Model file for the job. Use its own axes, mm. A direction names the side the tool comes from. Give positions to 0.01 mm unless a question says otherwise; leave off trailing zeros. Loops run counter-clockwise (first coordinate to the right, second up) from the corner with the lowest first, then second, coordinate; pieces in that order, holes last. Notation, with made-up numbers: M -2,23 L 38,23 A30 ccw 38,48 Z; hole C 50.25,-1.75 d8. An arc over 180 degrees is marked long. Use CSV: the item, a comma, the result in double quotes. Start each with the question number.
(1) Slice it at A-A on z = 20. State how many separate pieces and enclosed holes the cut face has, and give its area (3 significant figures).
(2) Wall check: line 1 along Y through (x, z) = (7, 2); line 2 along X through (y, z) = (11, 28); line 3 along Y through (x, z) = (0.7, 128.8). Give the ranges that are in metal, low to high. Write a range as from..to.
(3) Two-plate mould, pull along X, no slides. Class faces 1 (the face through (4, 7, 62)), 2 (the face through (37.14, 19.1, 1.52)), 3 (the face through (25.085, 15.049, 63.639)): pulls with the +X half, pulls with the -X half, needs draft (parallel to the pull), parting line crosses it, or undercut.
(4) Tool access for faces 4 (the face through (28.42, 6.35, 63.84)), 5 (the face through (6, 2, 3)), 6 (the face through (0.9, 19.14, 1.52)), 7 (the face through (12.724, 17.718, 62.16)): list every direction of +Z, -Z, +X, -X, +Y, -Y with a clear straight run to the whole face (end or side of a thin tool).
(5) Flat gauge pins, fed straight in: P1, Ø7.5, axis at x = 7, y = 4.5, coming from the +Z side; P2, Ø4, axis at x = 32, y = 29, coming from the -Z side; P3, Ø2.5, axis at y = -0.96, z = 128.8, coming from the +X side; P4, Ø1.5, axis at y = 3.5, z = 45.5, coming from the +X side. Where does each tip first touch, or does it go through?
(6) Slice it at B-B on y = 38.5. List the corners of the cut face in (x, z), and give its area (3 significant figures).
Autodesk Fusion 360 part; units mm, degrees
sketch "스케치1" plane through (0, 0, 0) normal (0, 0, 1) x (1, 0, 0)
  line L0 (0, 0) -> (38, 0)
  line L1 (38, 0) -> (38, 20)
  line L2 (38, 20) -> (0, 20)
  line L3 (0, 20) -> (0, 0)
  line L4 (0, 0) -> (0, 10)
  circle A0 centre (7, 16) radius 1.5
  circle A1 centre (31, 16) radius 1.5
  circle A2 centre (7, 4) radius 1.5
  circle A3 centre (31, 4) radius 1.5
  circle A4 centre (19, 10) radius 4
  line L5 (0, 10) -> (0, 13)
  line L6 (0, 13) -> (10, 13)
  line L7 (10, 13) -> (14.0415, 20)
  line L8 (10, 13) -> (18.0829, 13) construction
  line L9 (0, 10) -> (0, 7)
  line L10 (0, 10) -> (0, 7)
  line L11 (0, 7) -> (10, 7)
  line L12 (10, 7) -> (14.0311, 0.0179)
  line L13 (38, 10) -> (38, 13)
  line L14 (38, 13) -> (28, 13)
  line L15 (28, 13) -> (23.9585, 20)
  line L16 (28, 13) -> (36.0829, 13) construction
  line L17 (23.9585, 20) -> (14.0415, 20)
  line L18 (38, 10) -> (38, 7)
  line L19 (38, 7) -> (28, 7)
  line L20 (28, 7) -> (23.9585, 0)
  line L21 (28, 7) -> (36.0829, 7) construction
  line L22 (14.0415, 20) -> (23.9585, 20)
  line L23 (14.0311, 0.0179) -> (23.9585, 0)
  line L24 (27.134, 11.5) -> (23.0925, 18.5)
  line L25 (14.9075, 18.5) -> (23.0925, 18.5)
  line L26 (10.866, 11.5) -> (14.9075, 18.5)
  line L27 (1.5, 11.5) -> (10.866, 11.5)
  line L28 (1.5, 10) -> (1.5, 11.5)
  line L29 (1.5, 10) -> (1.5, 8.5)
  line L30 (1.5, 8.5) -> (10.866, 8.5)
  line L31 (10.866, 8.5) -> (14.8981, 1.5163)
  line L32 (14.8981, 1.5163) -> (23.0934, 1.5016)
  line L33 (27.134, 8.5) -> (23.0934, 1.5016)
  line L34 (36.5, 8.5) -> (27.134, 8.5)
  line L35 (36.5, 10) -> (36.5, 8.5)
  line L36 (36.5, 10) -> (36.5, 11.5)
  line L37 (36.5, 11.5) -> (27.134, 11.5)
  line L38 (19, 18.5) -> (20, 18.5)
  line L39 (19, 18.5) -> (18, 18.5)
  line L40 (18, 18.5) -> (17.9694, 1.5108)
  line L41 (20, 18.5) -> (19.9694, 1.5072)
  dimension "d1" = 38
  dimension "d2" = 20
  dimension "d7" = 3
  dimension "d8" = 3
  dimension "d9" = 3
  dimension "d10" = 3
  dimension "d11" = 8
  dimension "d12" = 3
  dimension "d13" = 10
  dimension "d14" = 60
  dimension "d15" = 120
  dimension "d16" = 10
  dimension "d17" = 120
  dimension "d19" = 10
  dimension "d20" = 120
  dimension "d21" = 1.5
  dimension "d22" = 1
  dimension "d23" = 1
extrude "돌출1" add sketch "스케치1" along normal blind 3 contours L0 L3 L4 L11 L12 L23 | L0 L1 L19 L20 | L1 L2 L3 L4 L5 L6 L7 L9 L10 L11 L12 L13 L14 L15 L17 L18 L19 L20 L22 L23 | L2 L3 L6 L7 | L1 L2 L14 L15 | A0 | A1 | A2 | A3 | A4 L41 | A4 L24 L25 L32 L33 L34 L35 L36 L37 L41 | A4 L40 L41 | A4 L25 L38 L39 L40 L41 | A4 L32 L40 L41 | A4 L40 | A4 L25 L26 L27 L28 L29 L30 L31 L32 L40 makes body 1
extrude "돌출2" add sketch "스케치1" against normal blind 2.5 contours A4 L41 | A4 L40 L41 | A4 L40 bodies 1
extrude "돌출3" cut sketch "스케치1" along normal blind 3 contours A0 | A1 | A2 | A3 bodies 1
extrude "돌출4" add sketch "스케치1" along normal blind 123 contours L1 L2 L3 L4 L5 L6 L7 L9 L10 L11 L12 L13 L14 L15 L17 L18 L19 L20 L22 L23 | A4 L40 L41 | A4 L25 L38 L39 L40 L41 | A4 L32 L40 L41 bodies 1
sketch "스케치2" plane through (0, 0, 123) normal (0, 0, 1) x (-1, 0, 0)
  line L0 (-36.5, -11.5) -> (-36.5, -8.5)
  line L1 (-36.5, -8.5) -> (-27.134, -8.5)
  line L2 (-27.134, -8.5) -> (-23.0934, -1.5016)
  line L3 (-23.0934, -1.5016) -> (-19.9694, -1.5072)
  line L4 (-19.9694, -1.5072) -> (-20, -18.5)
  line L5 (-20, -18.5) -> (-23.0925, -18.5)
  line L6 (-23.0925, -18.5) -> (-27.134, -11.5)
  line L7 (-27.134, -11.5) -> (-36.5, -11.5)
  line L8 (-1.5, -8.5) -> (-1.5, -11.5)
  line L9 (-1.5, -11.5) -> (-10.866, -11.5)
  line L10 (-10.866, -11.5) -> (-14.9075, -18.5)
  line L11 (-14.9075, -18.5) -> (-18, -18.5)
  line L12 (-18, -18.5) -> (-17.9694, -1.5108)
  line L13 (-17.9694, -1.5108) -> (-14.8981, -1.5163)
  line L14 (-14.8981, -1.5163) -> (-10.866, -8.5)
  line L15 (-10.866, -8.5) -> (-1.5, -8.5)
  line L16 (0, -13) -> (0, -7)
  line L17 (0, -7) -> (-10, -7)
  line L18 (-10, -7) -> (-14.0311, -0.0179)
  line L19 (-14.0311, -0.0179) -> (-23.9585, 0)
  line L20 (-23.9585, 0) -> (-28, -7)
  line L21 (-28, -7) -> (-38, -7)
  line L22 (-38, -7) -> (-38, -13)
  line L23 (-38, -13) -> (-28, -13)
  line L24 (-28, -13) -> (-23.9585, -20)
  line L25 (-23.9585, -20) -> (-14.0415, -20)
  line L26 (-14.0415, -20) -> (-10, -13)
  line L27 (-10, -13) -> (0, -13)
  line L28 (-18.9948, -0.0089) -> (-1.9949, -0.0396)
  line L29 (-1.9949, -0.0396) -> (-1.9859, 4.9604)
  line L30 (-1.9859, 4.9604) -> (-35.9859, 4.9604)
  line L31 (-35.9859, 4.9604) -> (-35.9859, -56.0396)
  line L32 (-35.9859, -56.0396) -> (-1.9859, -56.0396)
  line L33 (-1.9859, -56.0396) -> (-1.9859, 4.9604)
  line L34 (-35.9859, 4.9604) -> (-37.9859, 4.9604)
  line L35 (-1.9859, 4.9604) -> (0.0141, 4.9604)
  line L36 (0.0141, 4.9604) -> (0.0141, -56.0396)
  line L37 (0.0141, -56.0396) -> (-1.9859, -56.0396)
  line L38 (-1.9859, -56.0396) -> (-1.9859, 4.9604)
  line L39 (-37.9859, 4.9604) -> (-35.9859, 4.9604)
  line L40 (-35.9859, 4.9604) -> (-35.9859, -56.0396)
  line L41 (-35.9859, -56.0396) -> (-37.9859, -56.0396)
  line L42 (-37.9859, -56.0396) -> (-37.9859, 4.9604)
  line L43 (-1.9949, -0.0396) -> (-2.0309, -20.0395)
  line L44 (-2.0309, -20.0395) -> (-2.0309, -30.0395)
  line L45 (-2.0309, -30.0395) -> (-36.0309, -30.0395)
  line L46 (-35.9859, -56.0396) -> (-35.9859, -47.0396)
  line L47 (-35.9859, -47.0396) -> (-37.9859, -47.0396)
  line L48 (-35.9859, -47.0396) -> (0.0141, -47.0396)
  line L49 (-36.0309, -30.0395) -> (-38.0309, -30.0395)
  line L50 (-2.0309, -30.0395) -> (-0.0309, -30.0395)
  dimension "d32" = 17
  dimension "d33" = 5
  dimension "d34" = 34
  dimension "d35" = 61
  dimension "d36" = 2
  dimension "d37" = 2
  dimension "d38" = 61
  dimension "d39" = 20
  dimension "d40" = 10
  dimension "d41" = 34
  dimension "d56" = 9
  dimension "d57" = 36
  dimension "d60" = 2
  dimension "d61" = 2
extrude "돌출5" add sketch "스케치2" along normal blind 3 separate body contours L0 L1 L7 L21 L23 L31 L40 L42 | L0 L1 L7 L31 L40 | L1 L2 L3 L4 L5 L6 L7 L31 L40 | L1 L2 L3 L4 L5 L6 L7 L9 L10 L11 L12 L13 L14 L15 L17 L18 L19 L20 L21 L23 L24 L25 L26 L27 L28 L31 L40 L43 | L23 L31 L40 L42 L45 L49 | L23 L24 L25 L26 L27 L31 L40 L43 L44 L45 | L19 L20 L21 L28 L29 L30 L31 L40 | L21 L31 L34 L39 L40 L42 | L31 L33 L38 L40 L45 L48 L50 | L31 L40 L42 L45 L47 L49 | L31 L32 L33 L38 L40 L46 L48 | L31 L40 L41 L42 L46 L47 | L27 L33 L38 L43 L44 L50 | L16 L17 L27 L33 L35 L36 L38 L48 | L33 L36 L37 L38 L48 | L17 L18 L28 L43 | L8 L9 L15 L16 L17 L27 L33 L38 | L8 L9 L15 L33 L38 | L9 L10 L11 L12 L13 L14 L15 L43 makes body 2
extrude "돌출6" cut sketch "스케치2" along normal blind 3 contours L31 L33 L38 L40 L45 L48 L50 | L31 L32 L33 L38 L40 L46 L48 | L27 L33 L38 L43 L44 L50 bodies 2
sketch "스케치3" plane through (37.9859, 0, 0) normal (1, 0, 0) x (0, 1, 0)
  line L0 (-4.9604, 123) -> (56.0396, 123)
  line L1 (56.0396, 123) -> (56.0396, 126)
  line L2 (56.0396, 126) -> (-4.9604, 126)
  line L3 (-4.9604, 126) -> (-4.9604, 123)
  line L4 (-4.9604, 126) -> (-4.9604, 131)
  line L5 (-4.9604, 126) -> (-4.9604, 128.8)
  line L6 (-4.9604, 131) -> (56.0396, 131)
  line L7 (56.0396, 131) -> (56.0396, 126)
  line L8 (56.0396, 126) -> (-4.9604, 126)
  line L9 (-4.9604, 126) -> (-4.9604, 131)
  line L10 (-4.9604, 128.8) -> (56.0396, 128.8)
  line L11 (-4.9604, 128.8) -> (-0.9604, 128.8)
  line L12 (-0.9604, 128.8) -> (21.0396, 128.8)
  line L13 (21.0396, 128.8) -> (43.0396, 128.8)
  circle A0 centre (-0.9604, 128.8) radius 1.3
  circle A1 centre (21.0396, 128.8) radius 1.3
  circle A2 centre (43.0396, 128.8) radius 1.3
  line L14 (43.0396, 128.8) -> (47.0396, 128.8)
  line L15 (47.0396, 128.8) -> (47.0396, 131)
  line L16 (47.0396, 128.8) -> (47.0396, 126)
  line L17 (-4.9604, 123) -> (30.0396, 123)
  line L18 (30.0396, 123) -> (35.2357, 126)
  line L19 (30.0396, 123) -> (36.0396, 123) construction
  dimension "d46" = 5
  dimension "d47" = 2.8
  dimension "d48" = 61
  dimension "d49" = 4
  dimension "d50" = 22
  dimension "d51" = 22
  dimension "d52" = 2.6
  dimension "d53" = 2.6
  dimension "d54" = 2.6
  dimension "d55" = 4
  dimension "d62" = 35
  dimension "d63" = 30
extrude "돌출7" cut sketch "스케치2" along normal blind 3 contours L31 L32 L33 L38 L40 L46 L48 | L31 L40 L41 L42 L46 L47 | L33 L36 L37 L38 L48 bodies 2
extrude "돌출8" add sketch "스케치3" against normal blind 2 separate body contours L2 L4 L5 L8 L9 L10 L11 L12 L13 A0 A1 A2 L14 L16 | L4 L6 L9 L10 L11 L12 L13 A0 A1 A2 L14 L15 makes body 3
copy_body "CopyPasteBodies1" bodies 3 makes body 4
move_body "이동1" bodies 4 to x (1, 0, 0) y (0, 1, 0) z (0, 0, 1) at (-36, 0, 0)
extrude "돌출9" cut sketch "스케치3" against normal blind 38 contours L0 L1 L2 L8 L18 bodies 2
extrude "돌출10" cut sketch "스케치2" along normal blind 3 contours L1 L2 L3 L4 L5 L6 L7 L31 L40 | L9 L10 L11 L12 L13 L14 L15 L43 bodies 2
thread "스레드1"
thread "스레드2"
thread "스레드3"
thread "스레드4"
extrude "돌출11" cut 1 faces at (20.2188, 8.8691, -2.5) along direction (0, 0, 1) blind 2.5 on bodies 1 bodies 1
thread "스레드5"
thread "스레드6"
thread "스레드7"
thread "스레드8"
thread "스레드9"
thread "스레드10"
fillet "모깎기1" radius 3 4 edges at (38, 0, 1.5) (38, 20, 1.5) (0, 0, 1.5) (0, 20, 1.5) on bodies 1
fillet "모깎기2" radius 5 4 edges at (28, 13, 63) (10, 13, 63) (10, 7, 63) (28, 7, 63) on bodies 1
combine "결합1" operation add target body 1 tool bodies 3 2 4
fillet "모깎기3" radius 2 4 edges at (0.9859, -4.9604, 131) (36.9859, -4.9604, 131) (0.9859, 47.0396, 131) (36.9859, 47.0396, 131) on bodies 1
Reply:
1,separate pieces,"1"
1,enclosed holes,"2"
1,area,"187 mm^2"
2,line 1,"y = 0..2.5, 5.5..14.5, 17.5..20"
2,line 2,"x = 0..1.5, 17.99..19.99, 36.5..38"
2,line 3,"y = -4.96..-2.26, 0.34..19.74, 22.34..41.74, 44.34..47.04"
3,face 1,"needs draft"
3,face 2,"pulls with the +X half"
3,face 3,"undercut"
4,face 4,"+X, -Y"
4,face 5,"-X, -Y"
4,face 6,"-Z, -X, +Y"
4,face 7,"-X, +Y"
5,P1,"stops at z = 126"
5,P2,"stops at z = 123"
5,P3,"passes through"
5,P4,"stops at x = 26.41"
6,outline,"M -0.01,126 L 1.99,126 L 1.99,131 L -0.01,131 Z; M 35.99,126 L 37.99,126 L 37.99,131 L 35.99,131 Z"
6,area,"20.0 mm^2"
